Here's how the part is built. I have some questions about the finished solid (model axes, mm). Face numbers are marked on the shaded views. A direction names the side the tool comes from. Coordinates: 2 decimals unless noted, no trailing zeros. Write each loop counter-clockwise with the first axis right and the second up, starting at its lowest first coordinate (ties: lowest second). Pieces come first, ordered by that corner, then holes. Notation, with made-up numbers: (70, -37) -> (79, -37) arc R28 cw to (79, 2) -> close; hole circle Ø3 at (51, 79). An arc over 180 degrees is marked (long way). Use a Markdown table: item, result. Add a question column.
Item 1: Imagine slicing it at B-B, the plane x = 6.5. Write out the boundary of the cut face in (y, z).
Item 2: Imagine slicing it at C-C, the plane z = 11. Write out the boundary of the cut face in (x, y).
Item 3: On a 3-axis mill with a long thin cutter (end or side, diameter ignored), from which of +Z, -Z, +X, -X, +Y, -Y can I reach the whole of each face in a straight line? I mean the marked faces 1 and 2. Say none if no direction works.
Item 4: If I drill on line 1 along X through (y, z) = (8, 19); line 2 along Z through (x, y) = (22.5, 10.75); line 3 along Z through (x, y) = (2, 2.25), over which ranges is the centre line in solid material (lowest first)? Write a range as from..to.
Item 5: Imagine slicing it at D-D, the plane x = 27. Write out the boundary of the cut face in (y, z).
Item 6: Will these pins go through, and if not, where does the flat tip stop? pin 1 Ø1.5 at (x, z) = (27, 7.5) entering from -Y; pin 2 Ø3 at (x, y) = (32.5, -6) entering from +Z; pin 3 Ø3 at (x, y) = (22.5, 9.5) entering from -Z; pin 4 Ø6 at (x, y) = (9, -4.5) entering from +Z.
Item 7: Imagine slicing it at A-A, the plane y = 0. Write out the boundary of the cut face in (x, z), and give its area (3 significant figures).
```python
from build123d import *

# Parameters (mm, degrees)
F0_R     = 12.7
F1_DEPTH = 12.7
F2_W     = 25.4
F2_H     = 12.621605
F3_DEPTH = 38.1
F4_W     = 25.4
F4_H     = 6.35
F5_DEPTH = 51.562


with BuildPart() as f1:
    # F0 (on Right) → F1 (new body)
    with BuildSketch(Plane.YZ):
        with Locations((0, 12.621605)):
            Circle(F0_R)
    extrude(amount=F1_DEPTH)

    # F2 (on Right) → F3 (join)
    with BuildSketch(Plane.YZ):
        with Locations((0, 6.310802)):
            Rectangle(F2_W, F2_H)
    extrude(amount=F3_DEPTH)

    # F4 (on Front) → F5 (cut, symmetric)
    with BuildSketch(Plane.XZ):
        with Locations((25.4, 9.446605)):
            Rectangle(F4_W, F4_H)
    extrude(amount=F5_DEPTH, both=True, mode=Mode.SUBTRACT)


solid = f1.part
```
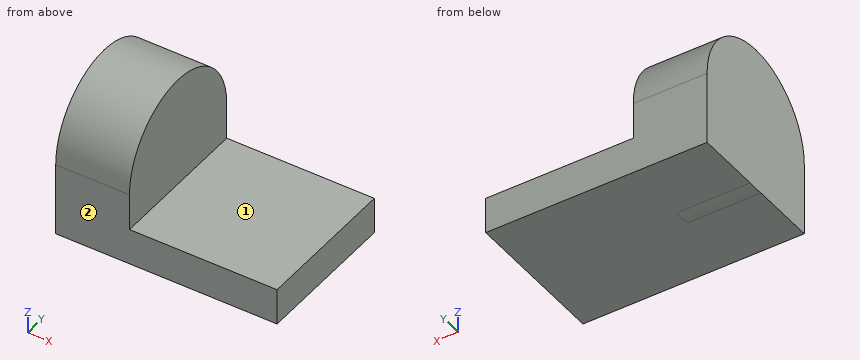
Ans:
| question | item | result |
|---|---|---|
| 1 | outline | (-12.7, 0) -> (-1.41, 0) arc R12.7 ccw to (1.41, 0) -> (12.7, 0) -> (12.7, 12.62) arc R12.7 ccw to (-12.7, 12.62) -> close |
| 2 | outline | (0, -12.7) -> (12.7, -12.7) -> (12.7, 12.7) -> (0, 12.7) -> close |
| 3 | face 1 | +Z, +X, +Y, -Y |
| 3 | face 2 | +Z, -Z, +X, -X, -Y |
| 4 | line 1 | x = 0..12.7 |
| 4 | line 2 | z = 0..6.27 |
| 4 | line 3 | z = 0..25.12 |
| 5 | outline | (-12.7, 0) -> (12.7, 0) -> (12.7, 6.27) -> (-12.7, 6.27) -> close |
| 6 | pin 1 | passes through |
| 6 | pin 2 | stops at z = 6.27 |
| 6 | pin 3 | stops at z = 0 |
| 6 | pin 4 | stops at z = 25.23 |
| 7 | outline | (0, -0.08) -> (12.7, -0.08) -> (12.7, 0) -> (38.1, 0) -> (38.1, 6.27) -> (12.7, 6.27) -> (12.7, 25.32) -> (0, 25.32) -> close |
| 7 | area | 482 mm^2 |
